from build123d import *

# Parameters (mm, degrees)
PAD004_DEPTH     = 50
POCKET011_DEPTH  = 211.5
POCKET012_DEPTH  = 5
CHAMFER_SIZE     = 1
POCKET013_DEPTH  = 0.001
POCKET014_DEPTH  = 3
POCKET016_DEPTH  = 198.2
POCKET017_DEPTH  = 201.2
SKETCH025_W      = 30
SKETCH025_H      = 5
POCKET019_DEPTH  = 3.55
PAD006_DEPTH     = 0.5
SKETCH026_R      = 2.55
PAD007_DEPTH     = 3
PAD008_DEPTH     = 1.5
SKETCH029_R      = 1.55
POCKET020_DEPTH  = 3.1
POCKET024_DEPTH  = 3
PAD011_DEPTH     = 1.5
PAD011_FACE129_W = 1
PAD011_FACE129_H = 10.802776
PAD012_DEPTH     = 1


with BuildPart() as part:
    # Sketch015 (on DatumPlane) → Pad004 (new body)
    with BuildSketch(Plane.XY.offset(-4.5)):
        with BuildLine():
            ThreePointArc((-100.8, 53.7125), (-102.426346, 53.038846), (-103.1, 51.4125))
            Line((-103.1, -51.4125), (-103.1, 51.4125))
            ThreePointArc((-103.1, -51.4125), (-102.426346, -53.038846), (-100.8, -53.7125))
            Line((100.8, -53.7125), (-100.8, -53.7125))
            ThreePointArc((100.8, -53.7125), (102.426346, -53.038846), (103.1, -51.4125))
            Line((103.1, 51.4125), (103.1, -51.4125))
            ThreePointArc((103.1, 51.4125), (102.426346, 53.038846), (100.8, 53.7125))
            Line((-100.8, 53.7125), (100.8, 53.7125))
        make_face()
    extrude(amount=-PAD004_DEPTH)

    # Sketch016 (on DatumPlane) → Pocket011 (cut)
    with BuildSketch(Plane(origin=(-105.75, 0, -8.5), x_dir=(0, 1, 0), z_dir=(1, 0, 0))):
        Polygon((-56.3625, -1), (48.97941, -10.216223), (56.3625, -1), (56.3625, -121), (-56.3625, -121), align=None)
    extrude(amount=POCKET011_DEPTH, mode=Mode.SUBTRACT)

    # Sketch017 (on Face5 of Pocket011) → Pocket012 (cut)
    with BuildSketch(Plane(origin=(0, 53.7125, -4.5), x_dir=(-1, 0, 0), z_dir=(0, 1, 0))):
        with BuildLine():
            ThreePointArc((-4, -3.05), (-4.707107, -3.342893), (-5, -4.05))
            Line((-5, -6.05), (-5, -4.05))
            ThreePointArc((-5, -6.05), (-4.707107, -6.757107), (-4, -7.05))
            Line((4, -7.05), (-4, -7.05))
            ThreePointArc((4, -7.05), (4.707107, -6.757107), (5, -6.05))
            Line((5, -4.05), (5, -6.05))
            ThreePointArc((5, -4.05), (4.707107, -3.342893), (4, -3.05))
            Line((-4, -3.05), (4, -3.05))
        make_face()
    extrude(amount=-POCKET012_DEPTH, mode=Mode.SUBTRACT)

    # Chamfer
    chamfer_edges = [part.edges().sort_by_distance(p)[0] for p in [
        (-103.1, -1.216545, -14.324646),
        (0, 48.97941, -18.716223),
    ]]
    chamfer(chamfer_edges, length=CHAMFER_SIZE)

    # Sketch018 (on Face8 of Chamfer) → Pocket013 (cut)
    with BuildSketch(Plane(origin=(0, 53.7125, -4.5), x_dir=(-1, 0, 0), z_dir=(0, 1, 0))):
        with BuildLine():
            Line((5, -4.05), (97.5, -4.05))
            ThreePointArc((97.770583, -4.320583), (97.691331, -4.129252), (97.5, -4.05))
            Line((97.770583, -4.320583), (97.770583, -5.779417))
            ThreePointArc((97.5, -6.05), (97.691331, -5.970748), (97.770583, -5.779417))
            Line((97.5, -6.05), (5, -6.05))
            Line((5, -4.05), (5, -6.05))
        make_face()
        with BuildLine():
            ThreePointArc((-97.5, -4.05), (-97.853553, -4.196447), (-98, -4.55))
            Line((-98, -5.55), (-98, -4.55))
            ThreePointArc((-98, -5.55), (-97.853553, -5.903553), (-97.5, -6.05))
            Line((-5, -6.05), (-97.5, -6.05))
            Line((-5, -4.05), (-5, -6.05))
            Line((-97.5, -4.05), (-5, -4.05))
        make_face()
    extrude(amount=-POCKET013_DEPTH, mode=Mode.SUBTRACT)

    # Sketch019 (on DatumPlane) → Pocket014 (cut)
    with BuildSketch(Plane.XY.offset(-11.05)):
        with BuildLine():
            ThreePointArc((-100.8, 53.7125), (-102.426346, 53.038846), (-103.1, 51.4125))
            Line((-103.1, 0), (-103.1, 51.4125))
            Line((-100.1, 0), (-103.1, 0))
            Line((-100.1, 0), (-100.1, 50.7125))
            Line((100.1, 50.7125), (-100.1, 50.7125))
            Line((100.1, 50.7125), (100.1, 0))
            Line((103.1, 0), (100.1, 0))
            Line((103.1, 0), (103.1, 51.4125))
            ThreePointArc((103.1, 51.4125), (102.426346, 53.038846), (100.8, 53.7125))
            Line((-100.8, 53.7125), (100.8, 53.7125))
        make_face()
    extrude(amount=POCKET014_DEPTH, mode=Mode.SUBTRACT)

    # Sketch021 (on DatumPlane) → Pocket016 (cut)
    with BuildSketch(Plane.YZ.offset(-99.1)):
        Polygon((-51.7125, -7.925444), (48.666642, -16.707481), (49.7125, -15.401948), (49.7125, 8.5), (-51.7125, 8.5), align=None)
    extrude(amount=POCKET016_DEPTH, mode=Mode.SUBTRACT)

    # Sketch022 (on DatumPlane) → Pocket017 (cut)
    with BuildSketch(Plane.YZ.offset(-100.6)):
        Polygon((-51.7125, 1.5), (-51.7125, -7.925444), (-1.5, -12.318468), (-1.5, -6.55), (51.2125, -6.55), (51.2125, 1.5), align=None)
        Polygon((48.666642, -16.707481), (49.7125, -15.401948), (51.2125, -12.55), (1.14642, -12.55), align=None)
    extrude(amount=POCKET017_DEPTH, mode=Mode.SUBTRACT)

    # Sketch025 (on DatumPlane) → Pocket019 (cut)
    with BuildSketch(Plane.XY.offset(-4.5)):
        Polygon((69.6, 51.2125), (101.6, 51.2125), (101.6, 37.636452), (97.6, 37.636452), (97.6, 48.7125), (69.6, 48.7125), align=None)
        with Locations((-84.6, 49.7125)):
            Rectangle(SKETCH025_W, SKETCH025_H)
    extrude(amount=-POCKET019_DEPTH, mode=Mode.SUBTRACT)

    # Pocket019 Face29 → Pad006 (add)
    with BuildSketch(Plane(origin=(-99.6, 50.141819, -6.918979), x_dir=(0, -1, 0), z_dir=(1, 0, 0))):
        Polygon((-2.070681, -2.418979), (-1.070681, -2.418979), (-1.070681, -0.368979), (2.929319, -0.368979), (2.929319, 1.131021), (-0.570681, 1.131021), (-2.070681, 1.131021), align=None)
    extrude(amount=PAD006_DEPTH)

    # Sketch026 (on Face60 of Pad006) → Pad007 (join)
    with BuildSketch(Plane.XY.offset(-6.55)):
        with Locations((-99.55, 22)):
            Circle(SKETCH026_R)
        with Locations((-99.55, -50.1625)):
            Circle(SKETCH026_R)
        with Locations((0, -50.1625)):
            Circle(SKETCH026_R)
        with Locations((99.55, -50.1625)):
            Circle(SKETCH026_R)
        with Locations((99.55, 22)):
            Circle(SKETCH026_R)
        with Locations((38.1, 50.1625)):
            Circle(SKETCH026_R)
        with Locations((-38.1, 50.1625)):
            Circle(SKETCH026_R)
    extrude(amount=PAD007_DEPTH)

    # Sketch026 (on Face60 of Pad006) → Pad008 (join)
    with BuildSketch(Plane.XY.offset(-6.55)):
        with Locations((-99.55, 22)):
            Circle(SKETCH026_R)
        with Locations((-99.55, -50.1625)):
            Circle(SKETCH026_R)
        with Locations((0, -50.1625)):
            Circle(SKETCH026_R)
        with Locations((99.55, -50.1625)):
            Circle(SKETCH026_R)
        with Locations((99.55, 22)):
            Circle(SKETCH026_R)
        with Locations((38.1, 50.1625)):
            Circle(SKETCH026_R)
        with Locations((-38.1, 50.1625)):
            Circle(SKETCH026_R)
    extrude(amount=-PAD008_DEPTH)

    # Sketch029 (on Face97 of Pad008) → Pocket020 (cut)
    with BuildSketch(Plane.XY.offset(-3.55)):
        with Locations((99.55, 22)):
            Circle(SKETCH029_R)
        with Locations((99.55, -50.1625)):
            Circle(SKETCH029_R)
        with Locations((0, -50.1625)):
            Circle(SKETCH029_R)
        with Locations((38.1, 50.1625)):
            Circle(SKETCH029_R)
        with Locations((-38.1, 50.1625)):
            Circle(SKETCH029_R)
        with Locations((-99.55, 22)):
            Circle(SKETCH029_R)
        with Locations((-99.55, -50.1625)):
            Circle(SKETCH029_R)
    extrude(amount=-POCKET020_DEPTH, mode=Mode.SUBTRACT)

    # Sketch032 (on Face15 of Pocket020) → Pocket024 (cut)
    with BuildSketch(Plane(origin=(0, 53.7125, -4.5), x_dir=(-1, 0, 0), z_dir=(0, 1, 0))):
        with BuildLine():
            ThreePointArc((-4.5, -1.8), (-5.737437, -2.312563), (-6.25, -3.55))
            Line((-6.25, -6.55), (-6.25, -3.55))
            ThreePointArc((-6.25, -6.55), (-5.737437, -7.787437), (-4.5, -8.3))
            Line((4.5, -8.3), (-4.5, -8.3))
            ThreePointArc((4.5, -8.3), (5.737437, -7.787437), (6.25, -6.55))
            Line((6.25, -3.55), (6.25, -6.55))
            ThreePointArc((6.25, -3.55), (5.737437, -2.312563), (4.5, -1.8))
            Line((-4.5, -1.8), (4.5, -1.8))
        make_face()
    extrude(amount=-POCKET024_DEPTH, mode=Mode.SUBTRACT)

    # Sketch033 (on Face32 of Pocket024) → Pad011 (join)
    with BuildSketch(Plane(origin=(0, 51.2125, -4.5), x_dir=(1, 0, 0), z_dir=(0, -1, 0))):
        with BuildLine():
            ThreePointArc((-4.5, -1.8), (-4.967707, -1.863658), (-5.401388, -2.05))
            Line((-7.71753, -2.05), (-5.401388, -2.05))
            ThreePointArc((-4.5, 0), (-6.407551, -0.556048), (-7.71753, -2.05))
            Line((-4.5, 0), (4.5, 0))
            ThreePointArc((7.71753, -2.05), (6.407551, -0.556048), (4.5, 0))
            Line((5.401388, -2.05), (7.71753, -2.05))
            ThreePointArc((5.401388, -2.05), (4.967707, -1.863658), (4.5, -1.8))
            Line((4.5, -1.8), (-4.5, -1.8))
        make_face()
    extrude(amount=PAD011_DEPTH)

    # Pad011 Face129 → Pad012 (add)
    with BuildSketch(Plane(origin=(0, 50.2125, -6.55), x_dir=(0, 1, 0), z_dir=(0, 0, 1))):
        Rectangle(PAD011_FACE129_W, PAD011_FACE129_H)
    extrude(amount=PAD012_DEPTH)


solid = part.part
Source: CAD feature listing. Evaluate the final solid. Frame: model axes, mm. A direction names the side the tool comes from. Give positions to 0.01 mm unless a question says otherwise; leave off trailing zeros. Write each loop counter-clockwise with the first axis right and the second up, starting at its lowest first coordinate (ties: lowest second). Pieces come first, ordered by that corner, then holes. Notation, with made-up numbers: (88.25, -6.75) -> (120.25, -6.75) arc R24 ccw to (120.25, 20.25) -> close; hole circle Ø3 at (-14.75, -15.5). An arc over 180 degrees is marked (long way). Return JSON: item names as keys, results as strings. Group by question number.
1. Material intervals for line 1 (Y direction, x = 99.55, z = -5.75); line 2 (Y direction, x = 5, z = -7.75); line 3 (X direction, y = 45, z = -9), sorted ascending. Write a range as from..to.
2. Access query for faces 1 (the face through (-100.6, 31, -14)), 2 (the face through (89, 50, -8.05)), 3 (the face through (69, 51, -11.05)). Directions: +Z, -Z, +X, -X, +Y, -Y. A direction counts if a zero-diameter tool reaches every point of the face in a straight line with its end or side. Return the directions, or none.
3. Pin query (flat end, axial travel): pin 1 Ø1 at (x, y) = (23, -22.5) entering from -Z; pin 2 Ø1 at (x, y) = (97.5, 21.5) entering from -Z; pin 3 Ø3 at (x, y) = (-40.5, -3) entering from +Z; pin 4 Ø3.5 at (x, y) = (-99.5, 22) entering from +Z. Return the tip coordinate at first contact, or that it passes through.
4. Section C-C, the plane y = -13.5. Output: boundary loops of the cut face in (x, z).
5. Mould query, pull axis Y, two halves, no side actions, for faces 4 (the face through (-85, 52.212, -6)), 5 (the face through (1, -53.712, -7)), 6 (the face through (40, 50, -3.55)). Classes: +Y half, -Y half, draft (parallel to the pull), parting line (faces both ways), or undercut.
6. Section B-B, the plane x = -47.5. Output: boundary loops of the cut face in (y, z).
7. Section A-A, the plane x = -79. Output: boundary loops of the cut face in (y, z).
Determined:
{
 "1": {"line 1": "y = -53.71..-51.71, -48.61..-47.61, 19.45..20.45, 23.55..24.55, 51.21..53.71", "line 2": "y = -53.71..-51.71, 49.71..50.71", "line 3": "x = -100.1..-99.1, 99.1..100.1"},
 "2": {"face 1": "none", "face 2": "+Z", "face 3": "+X, +Y"},
 "3": {"pin 1": "stops at z = -12.51", "pin 2": "stops at z = -16.36", "pin 3": "stops at z = -12.06", "pin 4": "stops at z = -3.55"},
 "4": {"outline": "(-103.1, -12.25) -> (-102.1, -13.25) -> (102.1, -13.25) -> (103.1, -12.25) -> (103.1, -4.5) -> (100.6, -4.5) -> (100.6, -11.27) -> (-100.6, -11.27) -> (-100.6, -4.5) -> (-103.1, -4.5) -> close"},
 "5": {"face 4": "undercut", "face 5": "-Y half", "face 6": "draft"},
 "6": {"outline": "(-53.71, -8.73) -> (-52.72, -9.82) -> (47.98, -18.63) -> (49.6, -17.94) -> (53.71, -12.81) -> (53.71, -11.05) -> (50.71, -11.05) -> (50.71, -8.05) -> (53.71, -8.05) -> (53.71, -4.5) -> (51.21, -4.5) -> (51.21, -6.55) -> (49.71, -6.55) -> (49.71, -12.55) -> (51.21, -12.55) -> (49.71, -15.4) -> (48.67, -16.71) -> (-51.71, -7.93) -> (-51.71, -4.5) -> (-53.71, -4.5) -> close"},
 "7": {"outline": "(-53.71, -8.73) -> (-52.72, -9.82) -> (47.98, -18.63) -> (49.6, -17.94) -> (53.71, -12.81) -> (53.71, -11.05) -> (50.71, -11.05) -> (50.71, -8.05) -> (49.71, -8.05) -> (49.71, -12.55) -> (51.21, -12.55) -> (49.71, -15.4) -> (48.67, -16.71) -> (-51.71, -7.93) -> (-51.71, -4.5) -> (-53.71, -4.5) -> close; (52.21, -8.05) -> (53.71, -8.05) -> (53.71, -4.5) -> (52.21, -4.5) -> close"}
}
